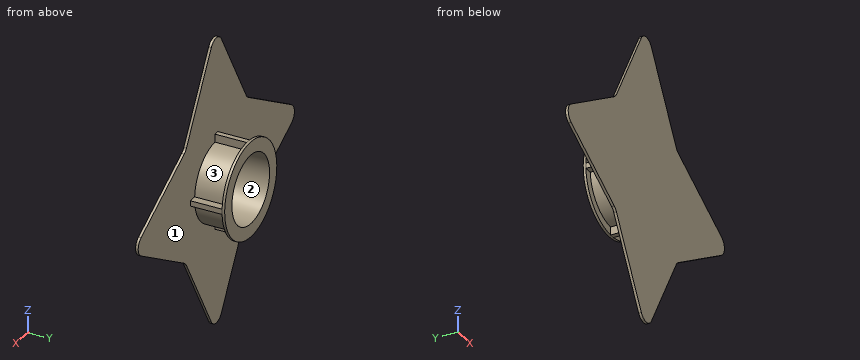
from build123d import *

# Parameters (mm, degrees)
EXTRUIR1_DEPTH = 5
REDONDEO1_R    = 20
EXTRUIR3_DEPTH = 60
CROQUIS4_R     = 90
EXTRUIR4_DEPTH = 5
CROQUIS5_R     = 65
EXTRUIR5_DEPTH = 65


with BuildPart() as part:
    # Croquis1 → Extruir1 (new body)
    with BuildSketch(Plane(origin=(0, 0, 0), x_dir=(1, 0, 0), z_dir=(0, 1, 0))):
        Polygon((106.066017178, 106.066017178), (289.777747887, 0), (106.066017178, -106.066017178), (0, -289.777747887), (-106.066017178, -106.066017178), (-289.777747887, 0), (-106.066017178, 106.066017178), (0, 289.777747887), align=None)
    extrude(amount=EXTRUIR1_DEPTH)

    # Redondeo1
    redondeo1_edges = [part.edges().sort_by_distance(p)[0] for p in [
        (106.066017178, 2.5, -106.066017178),
        (289.777747887, 2.5, 0),
        (106.066017178, 2.5, 106.066017178),
        (0, 2.5, 289.777747887),
        (-106.066017178, 2.5, 106.066017178),
        (-289.777747887, 2.5, 0),
        (-106.066017178, 2.5, -106.066017178),
        (0, 2.5, -289.777747887),
    ]]
    fillet(redondeo1_edges, radius=REDONDEO1_R)

    # Croquis2 → Extruir3 (add)
    with BuildSketch(Plane(origin=(0, 5, 0), x_dir=(1, 0, 0), z_dir=(0, 1, 0))):
        with BuildLine():
            Line((74.833147735, 5), (90, 5))
            Line((90, 5), (90, -5))
            Line((90, -5), (74.833147735, -5))
            ThreePointArc((74.833147735, -5), (53.033008589, -53.033008589), (5, -74.833147735))
            Line((5, -74.833147735), (5, -90))
            Line((5, -90), (-5, -90))
            Line((-5, -90), (-5, -74.833147735))
            ThreePointArc((-5, -74.833147735), (-53.033008589, -53.033008589), (-74.833147735, -5))
            Line((-74.833147735, -5), (-90, -5))
            Line((-90, -5), (-90, 5))
            Line((-90, 5), (-74.833147735, 5))
            ThreePointArc((-74.833147735, 5), (-53.033008589, 53.033008589), (-5, 74.833147735))
            Line((-5, 74.833147735), (-5, 90))
            Line((-5, 90), (5, 90))
            Line((5, 90), (5, 74.833147735))
            ThreePointArc((5, 74.833147735), (53.033008589, 53.033008589), (74.833147735, 5))
        make_face()
    extrude(amount=EXTRUIR3_DEPTH)

    # Croquis4 → Extruir4 (add)
    with BuildSketch(Plane(origin=(0, 65, 0), x_dir=(1, 0, 0), z_dir=(0, 1, 0))):
        with Locations(Location((0, 0, 0), (0, 0, 270))):
            Circle(CROQUIS4_R)
    extrude(amount=EXTRUIR4_DEPTH)

    # Croquis5 → Extruir5 (cut)
    with BuildSketch(Plane(origin=(0, 70, 0), x_dir=(1, 0, 0), z_dir=(0, 1, 0))):
        with Locations(Location((0, 0, 0), (0, 0, 270))):
            Circle(CROQUIS5_R)
    extrude(amount=-EXTRUIR5_DEPTH, mode=Mode.SUBTRACT)


solid = part.part
CAD build for the part. Positions are in the model's coordinates, mm. Face numbers are marked on the shaded views. Coordinates: 2 decimals unless noted, no trailing zeros. Write each loop counter-clockwise with the first axis right and the second up, starting at its lowest first coordinate (ties: lowest second). Pieces come first, ordered by that corner, then holes. Notation, with made-up numbers: (-10.75, 15) - (41.25, 15) arc R11 cw to (41.25, 30) - close; hole circle Ø11 at (29.25, 30.5). An arc over 180 degrees is marked (long way). Use a Markdown table: item, result. Add a question column.
Item 1: Band-saw the part on A-A, the plane y = 32. Give the cut face in (x, z), and give its area (3 significant figures).
Item 2: Band-saw the part on C-C, the plane x = -223. Give the cut face in (y, z), and give its area (3 significant figures).
Item 3: Mould opens along X. For the marked faces 1, 2 and 3 say: pulls with the +X half, pulls with the -X half, needs draft (parallel to the pull), parting line crosses it, or undercut.
Item 4: Flat gauge pins, fed straight in: pin 1 (5 mm diameter, centred on y = 44.5, z = 2, fed in from -X); pin 2 (11 mm diameter, centred on x = 2, y = 20, fed in from +Z); pin 3 (4 mm diameter, centred on y = 51.5, z = 55, fed in from -X); pin 4 (2 mm diameter, centred on x = 60.5, z = 91, fed in from -Y). Where does each tip first touch, or does it go through?
Item 5: Band-saw the part on B-B, the plane z = -118. Give the cut face in (x, y), and give its area (3 significant figures).
Item 6: Drill centre lines: L1, parallel to X at y = 24, z = 0; L2, parallel to Z at x = -40, y = 14.5; L3, parallel to Z at x = 17, y = 31. Where is each one in solid material? Low to high. Write a range as from..to.
Numbers:
| question | item | result |
|---|---|---|
| 1 | outline | (-90, -5) - (-74.83, -5) arc R75 ccw to (-5, -74.83) - (-5, -90) - (5, -90) - (5, -74.83) arc R75 ccw to (74.83, -5) - (90, -5) - (90, 5) - (74.83, 5) arc R75 ccw to (5, 74.83) - (5, 90) - (-5, 90) - (-5, 74.83) arc R75 ccw to (-74.83, 5) - (-90, 5) - close; hole circle Ø130 at (0, 0) |
| 1 | area | 5,000 mm2 |
| 2 | outline | (0, -38.55) - (5, -38.55) - (5, 38.55) - (0, 38.55) - close |
| 2 | area | 386 mm2 |
| 3 | face 1 | needs draft |
| 3 | face 2 | undercut |
| 3 | face 3 | pulls with the +X half |
| 4 | pin 1 | x = -90 |
| 4 | pin 2 | z = 90 |
| 4 | pin 3 | x = -53.07 |
| 4 | pin 4 | y = 0 |
| 5 | outline | (-99.18, 0) - (99.18, 0) - (99.18, 5) - (-99.18, 5) - close |
| 5 | area | 992 mm2 |
| 6 | L1 | -90..-65, 65..90 |
| 6 | L2 | -63.44..-51.23, 51.23..63.44 |
| 6 | L3 | -73.05..-62.74, 62.74..73.05 |
